```python
from build123d import *

# Parameters (mm, degrees)
SKETCH1_R           = 3
SKETCH1_R_2         = 0.75
BOSS_EXTRUDE1_DEPTH = 3
SKETCH2_R           = 2.5
SKETCH2_R_2         = 1.2
CUT_EXTRUDE1_DEPTH  = 0.3
CUT_EXTRUDE2_START  = -3
SKETCH2_2_R         = 2.5
SKETCH2_2_R_2       = 1.2
CUT_EXTRUDE2_DEPTH  = 0.3


with BuildPart() as part:
    # Sketch1 → Boss-Extrude1 (new body)
    with BuildSketch(Plane.XY):
        Circle(SKETCH1_R)
        Circle(SKETCH1_R_2, mode=Mode.SUBTRACT)
    extrude(amount=BOSS_EXTRUDE1_DEPTH)

    # Sketch2 → Cut-Extrude1 (cut)
    with BuildSketch(Plane.XY.offset(3)):
        Circle(SKETCH2_R)
        Circle(SKETCH2_R_2, mode=Mode.SUBTRACT)
    extrude(amount=-CUT_EXTRUDE1_DEPTH, mode=Mode.SUBTRACT)

    # Sketch2<2> → Cut-Extrude2 (cut)
    with BuildSketch(Plane.XY.offset(3).offset(CUT_EXTRUDE2_START)):
        Circle(SKETCH2_2_R)
        Circle(SKETCH2_2_R_2, mode=Mode.SUBTRACT)
    extrude(amount=CUT_EXTRUDE2_DEPTH, mode=Mode.SUBTRACT)


solid = part.part
```
Read the model definition and answer for the solid it produces. Units are mm, in the model's axes. A direction names the side the tool comes from. Give positions to 0.01 mm unless a question says otherwise; leave off trailing zeros. Order: outer loops, then holes, each group sorted by start corner. A loop starts at its lowest first (then second) coordinate and runs counter-clockwise, first axis right, second up. Notation, with made-up numbers: (-12, 6) -> (42, 6) arc R30 ccw to (42, 30) -> close; hole circle Ø11 at (-38.5, 77.5). An arc over 180 degrees is marked (long way). One line per item, written item: value. Start each with the question number.
(1) A tool of negligible diameter and unlimited length cuts with its end or side. For faces 1 (the flat face through (-1, -1, 0.3)), 2 (the flat face through (0, -1, 3)), 3 (the flat face through (-1, -1, 2.7)), from which of +Z, -Z, +X, -X, +Y, -Y can it reach the whole face along a straight path? Write none if from no direction.
(2) For a pull along Y with two mould halves and no side action, classify faces 4 (the flat face through (-2, 2, 3)), 5 (the cylindrical face through (-3, 0, 1)), 6 (the cylindrical face through (-0.75, 0.03, 1.48)) as released by +Y, released by -Y, zero draft, split by the parting line, or undercut.
(3) The part is cut by section A-A (x = 0). Determine the outline of the cut face in (y, z).
(4) A flat-ended cylindrical pin translates along its axis: P1, Ø1, axis at y = -1, z = 1, coming from the +X side. Find the tip coordinate at first contact, or state that the pin passes through.
(5) Straight lines are drawn through the part: L1, parallel to Y at x = 0, z = 2.8; L2, parallel to Y at x = 0, z = 1.85; L3, parallel to Z at x = -0.85, y = 1.45. For each, find the intervals that lie inside material, in ascending order.
(6) The part is cut by section D-D (x = 1.5). Determine the outline of the cut face in (y, z), and give its area (3 significant figures).
(7) The part is cut by section C-C (z = 0.2). Determine the outline of the cut face in (x, y).
Taken from the geometry:
1. face 1: -Z
1. face 2: +Z, +X, -X, +Y, -Y
1. face 3: +Z
2. face 4: zero draft
2. face 5: split by the parting line
2. face 6: undercut
3. outline: (-3, 0) -> (-2.5, 0) -> (-2.5, 0.3) -> (-1.2, 0.3) -> (-1.2, 0) -> (-0.75, 0) -> (-0.75, 3) -> (-1.2, 3) -> (-1.2, 2.7) -> (-2.5, 2.7) -> (-2.5, 3) -> (-3, 3) -> close; (0.75, 0) -> (1.2, 0) -> (1.2, 0.3) -> (2.5, 0.3) -> (2.5, 0) -> (3, 0) -> (3, 3) -> (2.5, 3) -> (2.5, 2.7) -> (1.2, 2.7) -> (1.2, 3) -> (0.75, 3) -> close
4. P1: x = 2.96
5. L1: -3 to -2.5, -1.2 to -0.75, 0.75 to 1.2, 2.5 to 3
5. L2: -3 to -0.75, 0.75 to 3
5. L3: 0.3 to 2.7
6. outline: (-2.6, 0) -> (-2, 0) -> (-2, 0.3) -> (2, 0.3) -> (2, 0) -> (2.6, 0) -> (2.6, 3) -> (2, 3) -> (2, 2.7) -> (-2, 2.7) -> (-2, 3) -> (-2.6, 3) -> close
6. area: 13.2 mm^2
7. outline: circle Ø6 at (0, 0); circle Ø2.4 at (0, 0); hole circle Ø5 at (0, 0); hole circle Ø1.5 at (0, 0)
